Check sheet for the modelled part. Datum: model origin and axes. Units: mm. Face numbers are marked on the shaded views. A direction names the side the tool comes from. Give positions to 0.01 mm unless a question says otherwise; leave off trailing zeros. Loops run counter-clockwise (first coordinate to the right, second up) from the corner with the lowest first, then second, coordinate; pieces in that order, holes last. Notation, with made-up numbers: M 87,30 L 127,30 A27 cw 127,47 Z; hole C -1.5,81 d10. An arc over 180 degrees is marked long. Write each question's results on one line, items separated by ' | '. Start each with the question number.
1. Sectioned sample at A-A on x = -41.5. Record the cut outline in (y, z) (3 decimals), and give its area (3 significant figures).
2. Draft check along Z on the marked faces 1 and 2. Enter one of: pulls with the +Z half, pulls with the -Z half, needs draft (parallel to the pull), parting line crosses it, or undercut.
3. Go/stop test with flat-tipped pins: pin 1 (5.5 mm diameter, centred on y = 6.5, z = -31.19, fed in from -X); pin 2 (3 mm diameter, centred on y = 10, z = 49, fed in from +X); pin 3 (3 mm diameter, centred on y = 11, z = 49.5, fed in from -X); pin 4 (10.5 mm diameter, centred on x = -47.5, z = -54, fed in from +Y). Record where each tip stops, or that it passes through.
4. Tool access check on the marked faces 3, 4 and 5. Record the directions out of +Z, -Z, +X, -X, +Y, -Y that give a thin tool (end or side, any length) a straight path to the whole face; none if there is none.
5. Material ranges on line 1 along Z through (x, y) = (-5.5, 8); line 2 along Z through (x, y) = (-39, 7.5); line 3 along Z through (x, y) = (-42.5, 4.25), recorded low to high.
6. Sectioned sample at B-B on x = 12.5. Record the cut outline in (y, z) (3 decimals).
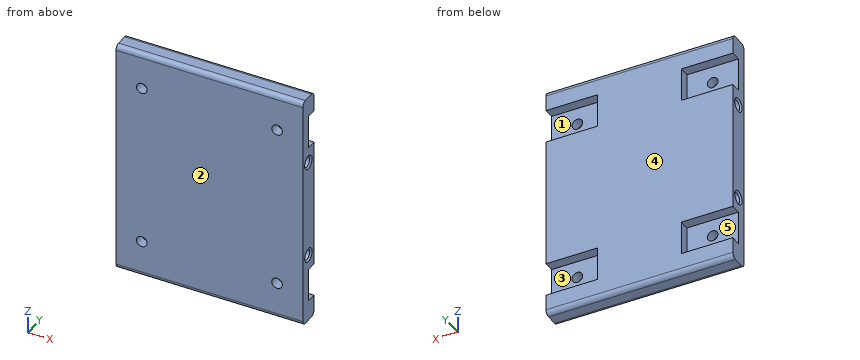
```python
from build123d import *

# Parameters (mm, degrees)
SKETCH1_W           = 117.7655389
SKETCH1_H           = 150
BOSS_EXTRUDE1_DEPTH = 13
FILLET1_R           = 3
SKETCH2_W           = 21.16486665
SKETCH2_H           = 6.5
CUT_EXTRUDE1_DEPTH  = 32.5
SKETCH3_R           = 3.35
CUT_EXTRUDE2_DEPTH  = 6.5
SKETCH4_R           = 3.325
CUT_EXTRUDE3_DEPTH  = 117.765539
CHAMFER1_SIZE       = 1


with BuildPart() as part:
    # Sketch1 → Boss-Extrude1 (new body)
    with BuildSketch(Plane(origin=(0, 0, 0), x_dir=(1, 0, 0), z_dir=(0, 1, 0))):
        Rectangle(SKETCH1_W, SKETCH1_H)
    extrude(amount=BOSS_EXTRUDE1_DEPTH)

    # Fillet1
    fillet1_edges = [part.edges().sort_by_distance(p)[0] for p in [
        (0, 13, 75),
        (0, 0, 75),
        (0, 0, -75),
        (0, 13, -75),
    ]]
    fillet(fillet1_edges, radius=FILLET1_R)

    # Sketch2 → Cut-Extrude1 (cut)
    with BuildSketch(Plane.ZY.offset(58.88276945)):
        with Locations((-51.59450088, 9.75)):
            Rectangle(SKETCH2_W, SKETCH2_H)
        with Locations((51.59450088, 9.75)):
            Rectangle(SKETCH2_W, SKETCH2_H)
    cut_extrude1 = extrude(amount=-CUT_EXTRUDE1_DEPTH, mode=Mode.SUBTRACT)

    # Sketch3 → Cut-Extrude2 (cut)
    with BuildSketch(Plane(origin=(0, 6.5, 0), x_dir=(1, 0, 0), z_dir=(0, 1, 0))):
        with Locations((-42.63276945, 51.59450088)):
            Circle(SKETCH3_R)
        with Locations((-42.63276945, -51.59450088)):
            Circle(SKETCH3_R)
    cut_extrude2 = extrude(amount=-CUT_EXTRUDE2_DEPTH, mode=Mode.SUBTRACT)

    # Mirror1: Cut-Extrude1, Cut-Extrude2 across plane
    add(cut_extrude1.mirror(Plane(origin=(0, 0, 0), x_dir=(0, 0, 1), z_dir=(1, 0, 0))), mode=Mode.SUBTRACT)
    add(cut_extrude2.mirror(Plane(origin=(0, 0, 0), x_dir=(0, 0, 1), z_dir=(1, 0, 0))), mode=Mode.SUBTRACT)

    # Sketch4 → Cut-Extrude3 (cut)
    with BuildSketch(Plane.ZY.offset(58.88276945)):
        with Locations((31.18900176, 6.5)):
            Circle(SKETCH4_R)
        with Locations((-31.18900176, 6.5)):
            Circle(SKETCH4_R)
    extrude(amount=-CUT_EXTRUDE3_DEPTH, mode=Mode.SUBTRACT)

    # Chamfer1
    chamfer1_edges = [part.edges().sort_by_distance(p)[0] for p in [
        (-58.88276945, 6.5, 27.86400176),
        (58.88276955, 6.5, 27.86400176),
        (-58.88276945, 6.5, -34.51400176),
        (58.88276955, 6.5, -34.51400176),
    ]]
    chamfer(chamfer1_edges, length=CHAMFER1_SIZE)


solid = part.part
```
Output values:
1) outline: M 0,-72 A3 ccw 3,-75 L 10,-75 A3 ccw 13,-72 L 13,-62.177 L 6.5,-62.177 L 6.5,-54.747 L 0,-54.747 Z; M 0,-48.442 L 6.5,-48.442 L 6.5,-41.012 L 13,-41.012 L 13,41.012 L 6.5,41.012 L 6.5,48.442 L 0,48.442 Z; M 0,54.747 L 6.5,54.747 L 6.5,62.177 L 13,62.177 L 13,72 A3 ccw 10,75 L 3,75 A3 ccw 0,72 Z; hole C 6.5,-31.189 d6.65; hole C 6.5,31.189 d6.65 | area: 1,520 mm2
2) face 1: undercut | face 2: needs draft
3) pin 1: through | pin 2: x = 26.38 | pin 3: x = -26.38 | pin 4: y = 6.5
4) face 3: +X, +Y | face 4: +Z, -Z, +X, -X, +Y | face 5: -X, +Y
5) line 1: -75 to -34.16, -28.22 to 28.22, 34.16 to 75 | line 2: -75 to -62.18, -41.01 to -34.36, -28.02 to 28.02, 34.36 to 41.01, 62.18 to 75 | line 3: -75 to -54.94, -48.25 to -33.64, -28.74 to 28.74, 33.64 to 48.25, 54.94 to 75
6) outline: M 0,-72 A3 ccw 3,-75 L 10,-75 A3 ccw 13,-72 L 13,72 A3 ccw 10,75 L 3,75 A3 ccw 0,72 Z; hole C 6.5,-31.189 d6.65; hole C 6.5,31.189 d6.65
